```python
from build123d import *

# Parameters (mm, degrees)
SALIENTE_EXTRUIR3_DEPTH = 80
CROQUIS2_R              = 2.35
CORTAR_EXTRUIR1_DEPTH   = 5
CORTAR_EXTRUIR2_START   = -5
CROQUIS3_R              = 2.35
CORTAR_EXTRUIR2_DEPTH   = 5
REDONDEO1_R             = 15
REDONDEO3_R             = 5


with BuildPart() as part:
    # Croquis1 → Saliente-Extruir3 (new body)
    with BuildSketch(Plane.XY):
        with BuildLine():
            Line((0, 0), (20, 0))
            ThreePointArc((20, 0), (27.071067812, -2.928932188), (30, -10))
            Line((30, -10), (30, -80))
            ThreePointArc((30, -80), (32.928932188, -87.071067812), (40, -90))
            Line((40, -90), (48, -90))
            Line((48, -90), (48, -100))
            Line((48, -100), (20, -100))
            Line((20, -100), (20, -10))
            Line((20, -10), (0, -10))
            Line((0, -10), (0, 0))
        make_face()
    extrude(amount=-SALIENTE_EXTRUIR3_DEPTH)

    # Croquis2 → Cortar-Extruir1 (cut)
    with BuildSketch(Plane.XY):
        with Locations((20, -5)):
            Circle(CROQUIS2_R)
    extrude(amount=-CORTAR_EXTRUIR1_DEPTH, mode=Mode.SUBTRACT)

    # Croquis3 → Cortar-Extruir2 (cut)
    with BuildSketch(Plane(origin=(0, 0, -80), x_dir=(-1, 0, 0), z_dir=(0, 0, -1)).offset(CORTAR_EXTRUIR2_START)):
        with Locations(Location((-20, -5, 0), (0, 0, 180))):
            Circle(CROQUIS3_R)
    extrude(amount=CORTAR_EXTRUIR2_DEPTH, mode=Mode.SUBTRACT)

    # Redondeo1
    redondeo1_edges = [part.edges().sort_by_distance(p)[0] for p in [
        (20, -100, -40),
    ]]
    fillet(redondeo1_edges, radius=REDONDEO1_R)

    # Redondeo3
    redondeo3_edges = [part.edges().sort_by_distance(p)[0] for p in [
        (20, -10, -40),
    ]]
    fillet(redondeo3_edges, radius=REDONDEO3_R)


solid = part.part
```
Read the model definition and answer for the solid it produces. Units are mm, in the model's axes. A direction names the side the tool comes from. Round coordinates to 2 decimals unless told otherwise and drop trailing zeros. Write each loop counter-clockwise with the first axis right and the second up, starting at its lowest first coordinate (ties: lowest second). Pieces come first, ordered by that corner, then holes. Notation, with made-up numbers: (-11, 80) - (20, 80) arc R13 ccw to (20, 105) - close; hole circle Ø1 at (29.25, 18.25). An arc over 180 degrees is marked (long way). One line per item, written item: value.
Q1. Straight lines are drawn through the part: line 1 (Y direction, x = 6.5, z = -36.5); line 2 (X direction, y = -79, z = -34); line 3 (Y direction, x = 46, z = -23.5). For each, find the intervals that lie inside material, in ascending order. Write a range as from..to.
The answers:
line 1: y = -10..0
line 2: x = 20..30
line 3: y = -100..-90
Q2. Find section D-D (y = -19). Determine the outline of the cut face in (x, z).
The answers:
outline: (20, -80) - (30, -80) - (30, 0) - (20, 0) - close
Q3. For a pull along X with two mould halves and no side action, classify faces 5 (the flat face through (20, -50, -39)), 6 (the flat face through (48, -95, -39)), 7 (the flat face through (20, -5, -5)), 8 (the flat face through (42, -100, -39)) as pulls with the +X half, pulls with the -X half, needs draft (parallel to the pull), parting line crosses it, or undercut.
The answers:
face 5: pulls with the -X half
face 6: pulls with the +X half
face 7: undercut
face 8: needs draft
Q4. Which of the six approach directions +Z, -Z, +X, -X, +Y, -Y give full straight-line access (tool end or side, diameter ignored) to faces 1 (the cylindrical face through (17.652, -4.897, -2.465)), 2 (the flat face through (44, -90, -39)), 3 (the cylindrical face through (17.652, -5.103, -77.465)), 4 (the flat face through (8, -10, -39))?
The answers:
face 1: +Z
face 2: +Z, -Z, +X, +Y
face 3: -Z
face 4: +Z, -Z, -X, -Y
Q5. Find section A-A (z = -66.5). Determine the outline of the cut face in (x, y).
The answers:
outline: (0, -10) - (15, -10) arc R5 cw to (20, -15) - (20, -85) arc R15 ccw to (35, -100) - (48, -100) - (48, -90) - (40, -90) arc R10 cw to (30, -80) - (30, -10) arc R10 ccw to (20, 0) - (0, 0) - close
Q6. Find section C-C (y = -5). Determine the outline of the cut face in (x, z), and give its area (3 significant figures).
The answers:
outline: (0, -80) - (17.65, -80) - (17.65, -75) - (22.35, -75) - (22.35, -80) - (28.66, -80) - (28.66, 0) - (22.35, 0) - (22.35, -5) - (17.65, -5) - (17.65, 0) - (0, 0) - close
area: 2,250 mm2
Q7. Find section B-B (x = 9). Determine the outline of the cut face in (y, z).
The answers:
outline: (-10, -80) - (0, -80) - (0, 0) - (-10, 0) - close
Q8. Each of these flat-tipped pins is pushed along its axis until it touches: P1, Ø1, axis at x = 37.5, z = -66.5, coming from the +Y side; P2, Ø6.5, axis at x = 44, z = -33.5, coming from the +Y side; P3, Ø10, axis at y = -77.5, z = -15, coming from the +X side. Where does it stop, or does it pass through?
The answers:
P1: stops at y = -89.54
P2: stops at y = -90
P3: stops at x = 30.32
